```python
from build123d import *

# Parameters (mm, degrees)
F1_DEPTH = 37.846
F3_DEPTH = 62.992
F4_R     = 8.427475
F5_DEPTH = 74.168


with BuildPart() as f1:
    # F0 (on Front) → F1 (new body, symmetric)
    with BuildSketch(Plane.XZ):
        Polygon((-47.176249, 47.191884), (-47.176249, 0), (33.306468, 0), (-8.186842, 47.191884), align=None)
    extrude(amount=F1_DEPTH, both=True)

    # F2 (on face) → F3 (cut)
    with BuildSketch(Plane.XZ.offset(37.846)):
        Polygon((-47.176249, 47.191884), (-47.176249, 39.384045), (-11.969197, 39.384045), (22.694981, 0), (33.306468, 0), (-8.186842, 47.191884), align=None)
    extrude(amount=-F3_DEPTH, mode=Mode.SUBTRACT)

    # F4 (on face) → F5 (cut)
    with BuildSketch(Plane(origin=(-47.176249, 0, 0), x_dir=(0, -1, 0), z_dir=(-1, 0, 0))):
        with Locations((0, 21.656843)):
            Circle(F4_R)
    extrude(amount=-F5_DEPTH, mode=Mode.SUBTRACT)


solid = f1.part
```
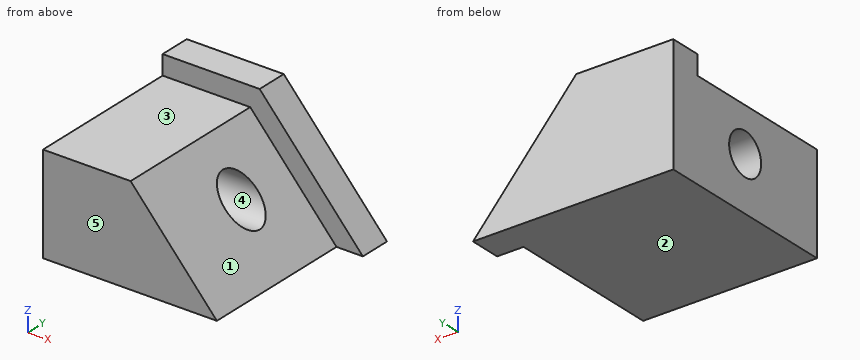
The listing builds one solid part. Answer for the finished solid, in the listing's coordinates (mm). Face numbers are marked on the shaded views. A direction names the side the tool comes from. Coordinates: 2 decimals unless noted, no trailing zeros. Write each loop counter-clockwise with the first axis right and the second up, starting at its lowest first coordinate (ties: lowest second). Pieces come first, ordered by that corner, then holes. Notation, with made-up numbers: (1.5, 1.25) - (6.5, 1.25) arc R11 cw to (6.5, 5.25) - close; hole circle Ø8 at (56.25, 48.25). An arc over 180 degrees is marked (long way). Return JSON: item names as keys, results as strings. Group by question number.
Q1. Flat-ended cylindrical pins translate along their axes: pin 1 Ø3 at (x, y) = (-18.5, -14.5) entering from +Z; pin 2 Ø8 at (x, z) = (24, 12.5) entering from -Y; pin 3 Ø13.5 at (y, z) = (0, 21.66) entering from +X; pin 4 Ø8 at (x, y) = (12, 7) entering from +Z. Find the tip coordinate at first contact, or state that the pin passes through.
Q2. Find the intervals of material crossed by line 1 along Z through (x, y) = (-30, 0); line 2 along Y through (x, z) = (-7, 16); line 3 along Z through (x, y) = (-40, -29), in increasing order. Write a range as [from, to].
Q3. The part is cut by section C-C on x = -30. Write down the section's boundary in (y, z), and give its area (3 significant figures).
Q4. Which of the six approach directions +Z, -Z, +X, -X, +Y, -Y give full straight-line access (tool end or side, diameter ignored) to the marked faces 1 and 2?
Q5. The part is cut by section A-A on z = 26. Write down the section's boundary in (x, y), and give its area (3 significant figures).
Q6. The part is cut by section B-B on y = 0. Write down the section's boundary in (x, z).
Q7. For a pull along Z with two mould halves and no side action, classify the marked faces 3, 4 and 5 as +Z half, -Z half, draft (parallel to the pull), parting line (faces both ways), or undercut.
Q8. The part is cut by section D-D on x = 8. Write down the section's boundary in (y, z), and give its area (3 significant figures).
Evaluation:
{
 "1": {"pin 1": "stops at z = 39.38", "pin 2": "stops at y = 25.15", "pin 3": "passes through", "pin 4": "stops at z = 16.7"},
 "2": {"line 1": "z = [0, 13.23], [30.08, 39.38]", "line 2": "y = [-37.85, -6.25], [6.25, 37.85]", "line 3": "z = [0, 39.38]"},
 "3": {"outline": "(-37.85, 0) - (37.85, 0) - (37.85, 47.19) - (25.15, 47.19) - (25.15, 39.38) - (-37.85, 39.38) - close; hole circle Ø16.85 at (0, 21.66)", "area": "2,860 mm2"},
 "4": {"face 1": "+Z, +X, -Y", "face 2": "-Z, +X, -X, +Y, -Y"},
 "5": {"outline": "(-47.18, -37.85) - (-0.19, -37.85) - (-0.19, -7.22) - (-47.18, -7.22) - close; (-47.18, 7.22) - (-0.19, 7.22) - (-0.19, 25.15) - (10.45, 25.15) - (10.45, 37.85) - (-47.18, 37.85) - close", "area": "3,010 mm2"},
 "6": {"outline": "(-47.18, 0) - (22.69, 0) - (11.05, 13.23) - (-47.18, 13.23) - close; (-47.18, 30.08) - (-3.78, 30.08) - (-11.97, 39.38) - (-47.18, 39.38) - close"},
 "7": {"face 3": "+Z half", "face 4": "undercut", "face 5": "draft"},
 "8": {"outline": "(-37.85, 0) - (37.85, 0) - (37.85, 28.78) - (25.15, 28.78) - (25.15, 16.7) - (6.81, 16.7) arc R8.43 cw to (-6.81, 16.7) - (-37.85, 16.7) - close", "area": "1,380 mm2"}
}
